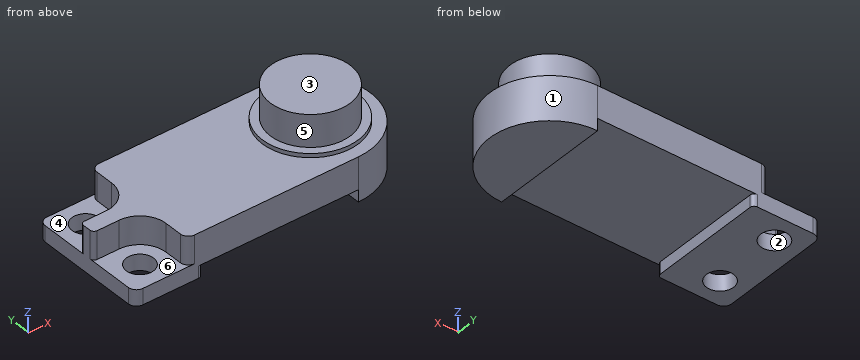
from build123d import *

# Parameters (mm, degrees)
EXTRUDE_1_DEPTH         = 5.5
SKETCH_2_W              = 19.5
SKETCH_2_H              = 1.5
CUT_EXTRUDE_1_DEPTH     = 32.372758884
SKETCH_3_W              = 6.5
SKETCH_3_H              = 3.5
CUT_EXTRUDE_2_DEPTH     = 6.5
SKETCH_4_W              = 3.5
SKETCH_4_H              = 6.5
CUT_EXTRUDE_3_DEPTH     = 6.5
HOLE_WIZARD_3_4_3_4_1_D = 3.4
FILLET_1_R              = 0.5
FILLET_2_R              = 1
FILLET_3_R              = 3.25


with BuildPart() as part:
    # 草图1 → 凸台-拉伸1 (new body)
    with BuildSketch(Plane.XY.offset(5.5)):
        with BuildLine():
            Line((19.5, 5.666127278), (-8.5, 5.666127278))
            Line((-8.5, 5.666127278), (-8.5, -9.333872722))
            Line((-8.5, -9.333872722), (19.5, -9.333872722))
            ThreePointArc((19.5, -9.333872722), (27, -1.833872722), (19.5, 5.666127278))
        make_face()
    extrude(amount=-EXTRUDE_1_DEPTH)

    # 草图2 → 切除-拉伸1 (cut, through all)
    with BuildSketch(Plane.XZ.offset(9.333872722)):
        with Locations((9.75, 0.75)):
            Rectangle(SKETCH_2_W, SKETCH_2_H)
    extrude(amount=-CUT_EXTRUDE_1_DEPTH, mode=Mode.SUBTRACT)

    # 草图3 → 切除-拉伸2 (cut)
    with BuildSketch(Plane(origin=(0, 5.666127278, 0), x_dir=(-1, 0, 0), z_dir=(0, 1, 0))):
        with Locations((5.25, 3.75)):
            Rectangle(SKETCH_3_W, SKETCH_3_H)
    extrude(amount=-CUT_EXTRUDE_2_DEPTH, mode=Mode.SUBTRACT)

    # 草图4 → 切除-拉伸3 (cut)
    with BuildSketch(Plane.ZY.offset(8.5)):
        with Locations((3.75, -6.083872722)):
            Rectangle(SKETCH_4_W, SKETCH_4_H)
    extrude(amount=-CUT_EXTRUDE_3_DEPTH, mode=Mode.SUBTRACT)

    # 草图5 → 旋转1 (revolve)
    with BuildSketch(Plane.XZ.offset(1.833872722), mode=Mode.PRIVATE) as revolve_1_sk:
        Polygon((24.49, 10), (19.5, 10), (19.5, 5.5), (25.5, 5.5), (25.5, 6), (24.49, 6), align=None)
    revolve(revolve_1_sk.sketch.rotate(Axis((19.5, -1.833872722, 10), (0, 0, -1)), 180), axis=Axis((19.5, -1.833872722, 10), (0, 0, -1)))

    # Ø3.4 (3.4) 直径孔1 (through all)
    with Locations(Plane.XY.offset(2)):
        with Locations((-5.25, 2.416127278), (-5.25, -6.083872722)):
            Hole(HOLE_WIZARD_3_4_3_4_1_D / 2)

    # 圆角1
    fillet_1_edges = [part.edges().sort_by_distance(p)[0] for p in [
        (0, 5.666127278, 0.75),
        (0, -9.333872722, 0.75),
        (-8.5, -0.833872722, 3.75),
        (-8.5, -2.833872722, 3.75),
    ]]
    fillet(fillet_1_edges, radius=FILLET_1_R)

    # 圆角2
    fillet_2_edges = [part.edges().sort_by_distance(p)[0] for p in [
        (-2, 5.666127278, 3.75),
        (-2, -9.333872722, 3.75),
        (-8.5, -9.333872722, 1),
        (-8.5, 5.666127278, 1),
    ]]
    fillet(fillet_2_edges, radius=FILLET_2_R)

    # 圆角3
    fillet_3_edges = [part.edges().sort_by_distance(p)[0] for p in [
        (-2, -0.833872722, 3.75),
        (-2, -2.833872722, 3.75),
    ]]
    fillet(fillet_3_edges, radius=FILLET_3_R)


solid = part.part
Can you work these out from the model? Positions are in its coordinate system, mm. Face numbers are marked on the shaded views. A direction names the side the tool comes from. Coordinates: 2 decimals unless noted, no trailing zeros. Write each loop counter-clockwise with the first axis right and the second up, starting at its lowest first coordinate (ties: lowest second). Pieces come first, ordered by that corner, then holes. Notation, with made-up numbers: (15, 8) -> (51, 8) arc R19 cw to (51, 44) -> close; hole circle Ø2 at (21.25, -19.75). An arc over 180 degrees is marked (long way). Answer as CSV lines item,"result".
1) If I drill on line 1 (Y direction, x = -5.25, z = 1.6); line 2 (X direction, y = -6.5, z = 0.75); line 3 (X direction, y = -2, z = 8.5), over which ranges is the centre line in solid material (lowest first)? Write a range as from..to.
Check result:
line 1,"-9.33..-7.78, -4.38..0.72, 4.12..5.67"
line 2,"-8.5..-6.9, -3.6..0, 19.5..25.37"
line 3,"14.51..24.49"
2) If we section it at C-C on z = 3: Please give me the cut outline in (x, y).
Check result:
outline,"(-8.5, -2.33) arc R0.5 ccw to (-8, -2.83) -> (-5.25, -2.83) arc R3.25 cw to (-2, -6.08) -> (-2, -8.33) arc R1 ccw to (-1, -9.33) -> (19.5, -9.33) arc R7.5 ccw to (19.5, 5.67) -> (-1, 5.67) arc R1 ccw to (-2, 4.67) -> (-2, 2.42) arc R3.25 cw to (-5.25, -0.83) -> (-8, -0.83) arc R0.5 ccw to (-8.5, -1.33) -> close"
3) If we mould it in two halves opening along Y, with no side actions, what happens to the marked faces 1, 2 and 3? For each: +Y half, -Y half, draft (parallel to the pull), parting line (faces both ways), or undercut.
Check result:
face 1,"parting line"
face 2,"undercut"
face 3,"draft"
4) If we section it at B-B on x = 23: Please give me the cut outline in (y, z), then the cut area to 3 significant figures.
Check result:
outline,"(-8.47, 0) -> (4.8, 0) -> (4.8, 5.5) -> (3.04, 5.5) -> (3.04, 6) -> (1.72, 6) -> (1.72, 10) -> (-5.39, 10) -> (-5.39, 6) -> (-6.71, 6) -> (-6.71, 5.5) -> (-8.47, 5.5) -> close"
area,"106 mm²"
5) If we section it at D-D on y = -7.25: Please give me the cut outline in (x, z), then the cut area to 3 significant figures.
Check result:
outline,"(-8.5, 0) -> (-6.49, 0) -> (-6.49, 2) -> (-8.5, 2) -> close; (-4.01, 0) -> (0, 0) -> (0, 1.5) -> (19.5, 1.5) -> (19.5, 0) -> (24.69, 0) -> (24.69, 5.5) -> (22.08, 5.5) -> (22.08, 6) -> (16.92, 6) -> (16.92, 5.5) -> (-2, 5.5) -> (-2, 2) -> (-4.01, 2) -> close"
area,"128 mm²"
6) On a 3-axis mill with a long thin cutter (end or side, diameter ignored), from which of +Z, -Z, +X, -X, +Y, -Y can I reach the whole of each face in a straight line? I mean the marked faces 4, 5 and 6. Say none if no direction works.
Check result:
face 4,"+Z, -X, +Y"
face 5,"+Z"
face 6,"+Z, -X, -Y"
7) If we section it at A-A on z = 1: Please give me the cut outline in (x, y).
Check result:
outline,"(-8.5, -8.33) arc R1 ccw to (-7.5, -9.33) -> (-0.5, -9.33) arc R0.5 ccw to (0, -8.83) -> (0, 5.17) arc R0.5 ccw to (-0.5, 5.67) -> (-7.5, 5.67) arc R1 ccw to (-8.5, 4.67) -> close; (19.5, -9.33) arc R7.5 ccw to (19.5, 5.67) -> close; hole circle Ø3.4 at (-5.25, -6.08); hole circle Ø3.4 at (-5.25, 2.42)"
8) Will these pins go through, and if not, where does the flat tip stop? P1, Ø3, axis at x = -5.25, y = -6.08, coming from the +Z side; P2, Ø1.8, axis at y = -7.5, z = 4, coming from the -X side; P3, Ø4.5, axis at x = 13.5, y = -4, coming from the -Z side; P4, Ø5.5, axis at x = -5, y = -6, coming from the +Z side.
Check result:
P1,"through"
P2,"x = -2"
P3,"z = 1.5"
P4,"z = 2"
